Input: part model. Units: mm. Frame: model coordinates. Coordinates: 2 decimals unless noted, no trailing zeros. Order: outer loops, then holes, each group sorted by start corner. A loop starts at its lowest first (then second) coordinate and runs counter-clockwise, first axis right, second up. Notation, with made-up numbers: M 25.5,8.25 L 63.5,8.25 A15 cw 63.5,19.25 Z; hole C 36,-26.5 d1. An arc over 180 degrees is marked long. Answer in a Markdown table with one row per item.
from build123d import *

# Parameters (mm, degrees)
SKETCH2_R           = 3.175
BOSS_EXTRUDE1_DEPTH = 3.175
SKETCH3_R           = 3.175
BOSS_EXTRUDE2_DEPTH = 14.351


with BuildPart() as part:
    # Sketch2 → Boss-Extrude1 (new body)
    with BuildSketch(Plane.XY.offset(17.526)):
        with BuildLine():
            ThreePointArc((238.125, 76.736249645), (225.425, 64.036249645), (238.125, 51.336249645))
            Line((238.125, 51.336249645), (242.474118596, 52.104143065))
            ThreePointArc((242.474118596, 52.104143065), (248.529898033, 56.754210308), (250.825, 64.036249645))
            ThreePointArc((250.825, 64.036249645), (248.529898033, 71.318288983), (242.474118596, 75.968356225))
            Line((242.474118596, 75.968356225), (238.125, 76.736249645))
        make_face()
        with Locations((238.125, 64.036249645)):
            Circle(SKETCH2_R, mode=Mode.SUBTRACT)
        with BuildLine():
            ThreePointArc((250.825, 64.036249645), (248.529898033, 56.754210308), (242.474118596, 52.104143065))
            Line((242.474118596, 52.104143065), (292.071750355, 60.861249645))
            ThreePointArc((292.071750355, 60.861249645), (288.896750355, 64.036249645), (292.071750355, 67.211249645))
            Line((292.071750355, 67.211249645), (242.474118596, 75.968356225))
            ThreePointArc((242.474118596, 75.968356225), (248.529898033, 71.318288983), (250.825, 64.036249645))
        make_face()
        with Locations((292.071750355, 64.036249645)):
            Circle(SKETCH2_R)
    boss_extrude1 = extrude(amount=-BOSS_EXTRUDE1_DEPTH)

    # Sketch3 → Boss-Extrude2 (add)
    with BuildSketch(Plane(origin=(0, 0, 14.351), x_dir=(-1, 0, 0), z_dir=(0, 0, -1))):
        with Locations((-292.071750355, 64.036249645)):
            Circle(SKETCH3_R)
    boss_extrude2 = extrude(amount=BOSS_EXTRUDE2_DEPTH)

    # Mirror1: Boss-Extrude1, Boss-Extrude2 across plane
    add(boss_extrude1.mirror(Plane.XY))
    add(boss_extrude2.mirror(Plane.XY))


solid = part.part
1) Cut plane D-D, the plane z = 13. Output: boundary loops of the cut face in (x, y) (3 decimals), and give its area (3 significant figures).
Resolved:
| item | result |
|---|---|
| outline | C 292.072,64.036 d6.35 |
| area | 31.7 mm2 |
2) Mould query, pull axis Y, two halves, no side actions, for faces 1 (the face through (225.43, 64.32, 15.96)), 2 (the face through (252, 64, -17.526)), 3 (the face through (235.8, 66.2, -16)). Classes: +Y half, -Y half, draft (parallel to the pull), parting line (faces both ways), or undercut.
Resolved:
| item | result |
|---|---|
| face 1 | parting line |
| face 2 | draft |
| face 3 | undercut |
3) Cut plane B-B, the plane x = 263.5. Output: boundary loops of the cut face in (y, z), and give its area (3 significant figures).
Resolved:
| item | result |
|---|---|
| outline | M 55.82,-17.53 L 72.26,-17.53 L 72.26,-14.35 L 55.82,-14.35 Z; M 55.82,14.35 L 72.26,14.35 L 72.26,17.53 L 55.82,17.53 Z |
| area | 104 mm2 |
4) Cut plane A-A, the plane y = 70.25. Output: boundary loops of the cut face in (x, z), and give its area (3 significant figures).
Resolved:
| item | result |
|---|---|
| outline | M 227.05,-17.53 L 274.86,-17.53 L 274.86,-14.35 L 227.05,-14.35 Z; M 227.05,14.35 L 274.86,14.35 L 274.86,17.53 L 227.05,17.53 Z |
| area | 304 mm2 |
5) Material intervals for probe 1 along Z at (x, y) = (265, 63); probe 2 along Y at (x, z) = (278, -15); probe 3 along X at (y, z) = (66.5, 10), sorted ascending.
Resolved:
| item | result |
|---|---|
| probe 1 | z = -17.53 to -14.35, 14.35 to 17.53 |
| probe 2 | y = 58.38 to 69.7 |
| probe 3 | x = 290.07 to 294.07 |
6) Cut plane C-C, the plane y = 65.25. Output: boundary loops of the cut face in (x, z).
Resolved:
| item | result |
|---|---|
| outline | M 225.48,-17.53 L 235.19,-17.53 L 235.19,-14.35 L 225.48,-14.35 Z; M 225.48,14.35 L 235.19,14.35 L 235.19,17.53 L 225.48,17.53 Z; M 241.06,-17.53 L 295.01,-17.53 L 295.01,17.53 L 241.06,17.53 L 241.06,14.35 L 289.14,14.35 L 289.14,-14.35 L 241.06,-14.35 Z |
